from build123d import *

# Parameters (mm, degrees)
SKETCH_2_R      = 1.5
SKETCH_2_R_2    = 2
SKETCH_2_W      = 42
SKETCH_2_H      = 22
SKETCH_2_R_3    = 1.6
EXTRUDE_2_DEPTH = 10
FILLET_1_R      = 2


with BuildPart() as part:
    # 草图2 → 凸台-拉伸2 (new body)
    with BuildSketch(Plane.XY):
        with BuildLine():
            ThreePointArc((35.709805767, -12.992681481), (37.684421913, 4.88716125), (31.214285714, 21.671833502))
            Line((31.214285714, 21.671833502), (32.857142857, 22.812456318))
            ThreePointArc((32.857142857, 22.812456318), (8.608258655, 39.062742901), (-20.224954765, 34.510160892))
            Line((-20.224954765, 34.510160892), (-17.696835419, 30.19639078))
            ThreePointArc((-17.696835419, 30.19639078), (-22.408690047, -26.885881246), (32.890610575, -11.96694347))
            Line((32.890610575, -11.96694347), (35.709805767, -12.992681481))
        make_face()
        with Locations((-19.798989873, -19.798989873)):
            Circle(SKETCH_2_R, mode=Mode.SUBTRACT)
        with Locations((0, -28)):
            Circle(SKETCH_2_R, mode=Mode.SUBTRACT)
        with Locations((-14.5, -5)):
            Circle(SKETCH_2_R_2, mode=Mode.SUBTRACT)
        with Locations((-28, 0)):
            Circle(SKETCH_2_R, mode=Mode.SUBTRACT)
        with Locations((19.798989873, -19.798989873)):
            Circle(SKETCH_2_R, mode=Mode.SUBTRACT)
        with Locations((10, 0)):
            Rectangle(SKETCH_2_W, SKETCH_2_H, mode=Mode.SUBTRACT)
        with Locations((34.5, -5)):
            Circle(SKETCH_2_R_2, mode=Mode.SUBTRACT)
        with Locations((-14.5, 5)):
            Circle(SKETCH_2_R_2, mode=Mode.SUBTRACT)
        with Locations((-19.798989873, 19.798989873)):
            Circle(SKETCH_2_R, mode=Mode.SUBTRACT)
        with Locations((0, 28)):
            Circle(SKETCH_2_R, mode=Mode.SUBTRACT)
        with Locations((19.798989873, 19.798989873)):
            Circle(SKETCH_2_R, mode=Mode.SUBTRACT)
        with Locations((34.5, 5)):
            Circle(SKETCH_2_R_2, mode=Mode.SUBTRACT)
        with Locations((26.516504294, 26.516504294)):
            Circle(SKETCH_2_R_3, mode=Mode.SUBTRACT)
        with Locations((14.350628714, 34.645482469)):
            Circle(SKETCH_2_R, mode=Mode.SUBTRACT)
        with Locations((0, 37.5)):
            Circle(SKETCH_2_R, mode=Mode.SUBTRACT)
        with Locations((-14.350628714, 34.645482469)):
            Circle(SKETCH_2_R, mode=Mode.SUBTRACT)
    extrude(amount=EXTRUDE_2_DEPTH)

    # 圆角1
    # the kernel refuses this fillet: 2 mm, written as the material it adds along each edge
    with BuildSketch(Plane(origin=(-17.696835419, 30.19639078, 0), x_dir=(-0.5056238691162223, 0.862754022291372, 0), z_dir=(0, 0, 1))) as fillet_1_piece_1:
        with BuildLine():
            CenterArc((1.945906404, 2), FILLET_1_R, 183.09857934, 86.90142066)
            ThreePointArc((-0.051169618, 1.891891892), (-0.012794743, 0.946291876), (0, 0))
            Line((0, 0), (1.945906404, 0))
        make_face()
    extrude(amount=10)
    # the kernel refuses this fillet: 2 mm, written as the material it takes off along each edge
    with BuildSketch(Plane(origin=(35.709805767, -12.992681481, -5.279816712), x_dir=(0.3156668887072375, 0.9488700729677867, 0), z_dir=(0, 0, 1))) as fillet_1_2_piece_1:
        with BuildLine():
            CenterArc((2.056349667, 1.99922765), FILLET_1_R, 178.407630732, 93.184738537)
            Line((0.057122017, 2.054804668), (0, 0))
            ThreePointArc((0, 0), (1.055963342, -0.014674657), (2.111926685, 0))
        make_face()
    extrude(amount=20.559633424, mode=Mode.SUBTRACT)
    with BuildSketch(Plane(origin=(32.857142857, 22.812456318, -5.26498253), x_dir=(-0.8214285714285717, -0.5703114079525466, 0), z_dir=(0, 0, 1))) as fillet_1_2_piece_2_section:
        with BuildLine():
            CenterArc((2.052668078, -2), FILLET_1_R, 90, 93.01696131)
            ThreePointArc((0.055440082, -2.105263158), (0.013862423, -1.052996506), (0, 0))
            Line((0, 0), (2.052668078, 0))
        make_face()
    fillet_1_2_piece_2 = extrude(amount=20.52996506, mode=Mode.PRIVATE)
    fillet_1_2_piece_2 = fillet_1_2_piece_2 - Plane(origin=(0, 0, 5), x_dir=(0.9397317307134324, -0.3419126705612664, 0), z_dir=(0, 0, -1)) * Cylinder(38, 50, mode=Mode.PRIVATE)
    add(fillet_1_2_piece_2, mode=Mode.SUBTRACT)
    with BuildSketch(Plane(origin=(-20.224954765, 34.510160892, -5.26498253), x_dir=(0.8757655299583756, 0.48273671554660663, 0), z_dir=(0, 0, 1))) as fillet_1_2_piece_3:
        with BuildLine():
            CenterArc((2.053343187, -1.999306879), FILLET_1_R, 88.491519345, 93.01696131)
            Line((0.054036308, -2.051956704), (0, 0))
            ThreePointArc((0, 0), (1.052996506, 0.013862423), (2.105993012, 0))
        make_face()
    extrude(amount=20.52996506, mode=Mode.SUBTRACT)


solid = part.part
Geometry: final body of the model. Coordinates: model frame, mm. A direction names the side the tool comes from. Coordinates: 2 decimals unless noted, no trailing zeros. Loops run counter-clockwise (first coordinate to the right, second up) from the corner with the lowest first, then second, coordinate; pieces in that order, holes last. Notation, with made-up numbers: (0.25, 21) - (6.25, 21) arc R23 cw to (6.25, 33) - close; hole circle Ø2 at (-17, -4.75). An arc over 180 degrees is marked (long way). One line per question, with ' | ' between items. Start each with the question number.
(1) Reachability of faces 1 (the flat face through (10, -11, 5)), 2 (the cylindrical face through (8.988, 38.977, 4.93)) from +Z, -Z, +X, -X, +Y, -Y: full face, straight path, thin tool, end or side. Return the list, or none.
(2) Draft query along X for faces 3 (the cylindrical face through (-0.195, -26.513, 4.93)), 4 (the flat face through (-11.3, 6.5, 10)), 5 (the cylindrical face through (-18.463, 30.391, 4.93)). Return one class per face: +X half, -X half, draft (parallel to the pull), parting line (faces both ways), or undercut.
(3) Cut plane D-D on x = -14.5. Output: boundary loops of the cut face in (y, z).
(4) Cut plane B-B on x = 0. Output: boundary loops of the cut face in (y, z), and give its area (3 significant figures).
(5) Cut plane C-C on y = 5. Output: boundary loops of the cut face in (x, z).
(6) Cut plane A-A on y = -28. Output: boundary loops of the cut face in (x, z).
(7) Ray query, L1, parallel to X at y = -0.5, z = 8; L2, parallel to Y at x = 14, z = 7; L3, parallel to Y at x = 1, z = 2.25. Return the intervals inside material, ascending. Write a range as from..to.
(8) First-contact query: pin 1 (5 mm diameter, centred on x = -28, y = 0, fed in from -Z); pin 2 (5 mm diameter, centred on x = 17.5, z = 5, fed in from -Y); pin 3 (3 mm diameter, centred on x = 16, z = 5, fed in from +Y); pin 4 (1 mm diameter, centred on x = -9.5, z = 8.5, fed in from +Y). Flat tips, straight axial feed; report the tip coordinate or a pass-through.
Here are the results:
1) face 1: +Z, -Z | face 2: +Z, -Z, +Y
2) face 3: undercut | face 4: draft | face 5: -X half
3) outline: (-31.86, 0) - (-7, 0) - (-7, 10) - (-31.86, 10) - close; (-3, 0) - (3, 0) - (3, 10) - (-3, 10) - close; (7, 0) - (33.15, 0) - (33.15, 10) - (7, 10) - close; (36.14, 0) - (37.28, 0) - (37.28, 10) - (36.14, 10) - close
4) outline: (-35, 0) - (-29.5, 0) - (-29.5, 10) - (-35, 10) - close; (-26.5, 0) - (-11, 0) - (-11, 10) - (-26.5, 10) - close; (11, 0) - (26.5, 0) - (26.5, 10) - (11, 10) - close; (29.5, 0) - (36, 0) - (36, 10) - (29.5, 10) - close; (39, 0) - (40, 0) - (40, 10) - (39, 10) - close | area: 440 mm²
5) outline: (-34.64, 0) - (-16.5, 0) - (-16.5, 10) - (-34.64, 10) - close; (-12.5, 0) - (-11, 0) - (-11, 10) - (-12.5, 10) - close; (31, 0) - (32.5, 0) - (32.5, 10) - (31, 10) - close; (36.5, 0) - (37.67, 0) - (37.67, 10) - (36.5, 10) - close
6) outline: (-21, 0) - (-1.5, 0) - (-1.5, 10) - (-21, 10) - close; (1.5, 0) - (21, 0) - (21, 10) - (1.5, 10) - close
7) L1: -35..-29.41, -26.59..-11, 31..38 | L2: -32.08..-11, 11..33.19, 36.1..37.47 | L3: -34.99..-29.12, -26.88..-11, 11..26.88, 29.12..36.38, 38.62..39.99
8) pin 1: z = 0 | pin 2: y = -31.62 | pin 3: y = 37.28 | pin 4: y = 38.97
